Read the model definition and answer for the solid it produces. Units are mm, in the model's axes. A direction names the side the tool comes from. Coordinates: 2 decimals unless noted, no trailing zeros. Loops run counter-clockwise (first coordinate to the right, second up) from the corner with the lowest first, then second, coordinate; pieces in that order, holes last. Notation, with made-up numbers: (53.5, 22.25) - (93.5, 22.25) arc R23 cw to (93.5, 40.25) - close; hole circle Ø6 at (66.25, 48). An arc over 180 degrees is marked (long way). Use one line per item in the form item = value. Start each with the question number.
1) Each of these flat-tipped pins is pushed along its axis until it touches: P1, Ø8, axis at x = -3, z = -5, coming from the -Y side; P2, Ø4, axis at x = -23.5, z = -11.5, coming from the +Y side; P3, Ø6, axis at x = 5.5, z = -5, coming from the +Y side. Where does it stop, or does it pass through?
2) A cutting plane is placed at D-D (z = 13). Give the vertices of the cut face in (x, y), and give its area (3 significant figures).
3) Consider line 1 (X direction, y = 13, z = -4); line 2 (Y direction, x = -5.5, z = 0) (3 decimals); line 3 (Z direction, x = 21, y = -3.5). Determine where each line is inside the solid, lowest interval first.
4) A cutting plane is placed at C-C (x = 27). Give the vertices of the cut face in (y, z) (3 decimals), and give its area (3 significant figures).
5) A cutting plane is placed at A-A (y = 0). Give the vertices of the cut face in (x, z) (3 decimals).
6) The mould has two halves that part along X. Classify faces 3 (the face through (38.1, 7, -7)), 4 (the face through (34.237, 14.647, 7.618)), 5 (the face through (-0.427, -7.296, -7.956)): released by +X, released by -X, zero draft, split by the parting line, or undercut.
7) Which of the six approach directions +Z, -Z, +X, -X, +Y, -Y give full straight-line access (tool end or side, diameter ignored) to faces 1 (the face through (-30.48, 11, -3)), 2 (the face through (-38.1, 7, 7))?
from build123d import *

# Parameters (mm, degrees)
SKETCH1_W = 30.48
SKETCH1_H = 1.27


with BuildPart() as part:
    # Sketch1 → Revolve2 (revolve)
    with BuildSketch(Plane.XY, mode=Mode.PRIVATE) as revolve2_sk:
        with Locations((15.24, 10.16)):
            Rectangle(SKETCH1_W, SKETCH1_H)
        with Locations((-15.24, 10.16)):
            Rectangle(SKETCH1_W, SKETCH1_H)
        Polygon((30.48, 10.795), (30.48, 9.525), (38.1, 9.525), (38.1, 16.51), (30.48, 16.51), align=None)
        Polygon((-38.1, 9.525), (-30.48, 9.525), (-30.48, 10.795), (-30.48, 16.51), (-38.1, 16.51), align=None)
    revolve(revolve2_sk.sketch.rotate(Axis((-30.48, 0, 0), (1, 0, 0)), 90), axis=Axis((-30.48, 0, 0), (1, 0, 0)))


solid = part.part
Found:
q1.P1 = -10.75
q1.P2 = 5.13
q1.P3 = 10.61
q2.outline = (-38.1, -10.18) - (-30.48, -10.18) - (-30.48, 10.18) - (-38.1, 10.18) - close; (30.48, -10.18) - (38.1, -10.18) - (38.1, 10.18) - (30.48, 10.18) - close
q2.area = 310 mm^2
q3.line_1 = -38.1 to -30.48, 30.48 to 38.1
q3.line_2 = -10.795 to -9.525, 9.525 to 10.795
q3.line_3 = -10.21 to -8.86, 8.86 to 10.21
q4.outline = circle Ø21.59 at (0, 0); hole circle Ø19.05 at (0, 0)
q4.area = 81.1 mm^2
q5.outline = (-38.1, -16.51) - (-30.48, -16.51) - (-30.48, -10.795) - (30.48, -10.795) - (30.48, -16.51) - (38.1, -16.51) - (38.1, -9.525) - (-38.1, -9.525) - close; (-38.1, 9.525) - (38.1, 9.525) - (38.1, 16.51) - (30.48, 16.51) - (30.48, 10.795) - (-30.48, 10.795) - (-30.48, 16.51) - (-38.1, 16.51) - close
q6.face_3 = released by +X
q6.face_4 = zero draft
q6.face_5 = undercut
q7.face_1 = none
q7.face_2 = +Z, -Z, -X, +Y, -Y
